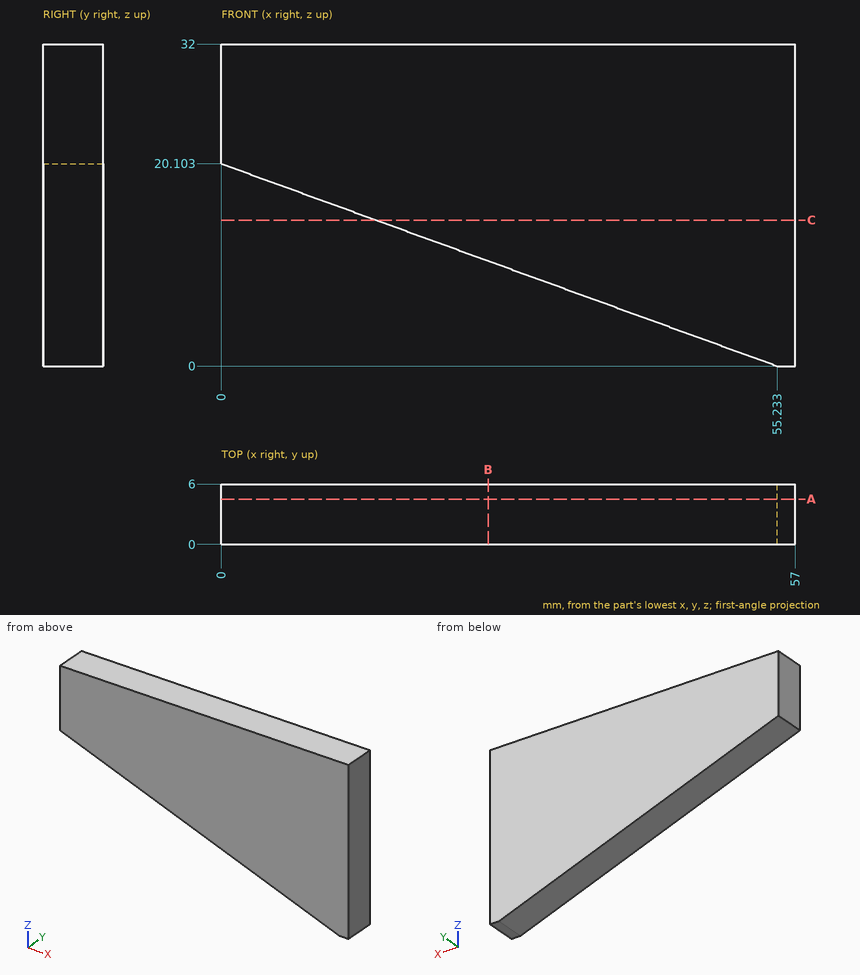
Drawing for the job (mm, zero at the part's lowest x, y, z). Give positions to 0.01 mm unless a question says otherwise; leave off trailing zeros. Loops run counter-clockwise (first coordinate to the right, second up) from the corner with the lowest first, then second, coordinate; pieces in that order, holes last.
1) Band-saw the part on C-C on z = 14.5. List the corners of the cut face in (x, y).
Values follow:
outline: (15.39, 0) - (57, 0) - (57, 6) - (15.39, 6) - close
2) Probe line 1 along Z through (x, y) = (28.5, 2.3); line 2 along Z through (x, y) = (20, 2.2). List the from-to ranges inside material, lowest first.
Values follow:
line 1: z = 9.73 to 32
line 2: z = 12.82 to 32
3) Drop a flat-ended pin along its axis: P1, Ø3, axis at x = 22.5, z = 28, coming from the -Y side. Give the stop position or say it passes through.
Values follow:
P1: stops at y = 0
4) Band-saw the part on A-A on y = 4.5. List the corners of the cut face in (x, z), then the cut area to 3 significant figures.
Values follow:
outline: (0, 20.1) - (55.23, 0) - (57, 0) - (57, 32) - (0, 32) - close
area: 1,270 mm2
5) Band-saw the part on B-B on x = 26.5. List the corners of the cut face in (y, z).
Values follow:
outline: (0, 10.46) - (6, 10.46) - (6, 32) - (0, 32) - close
